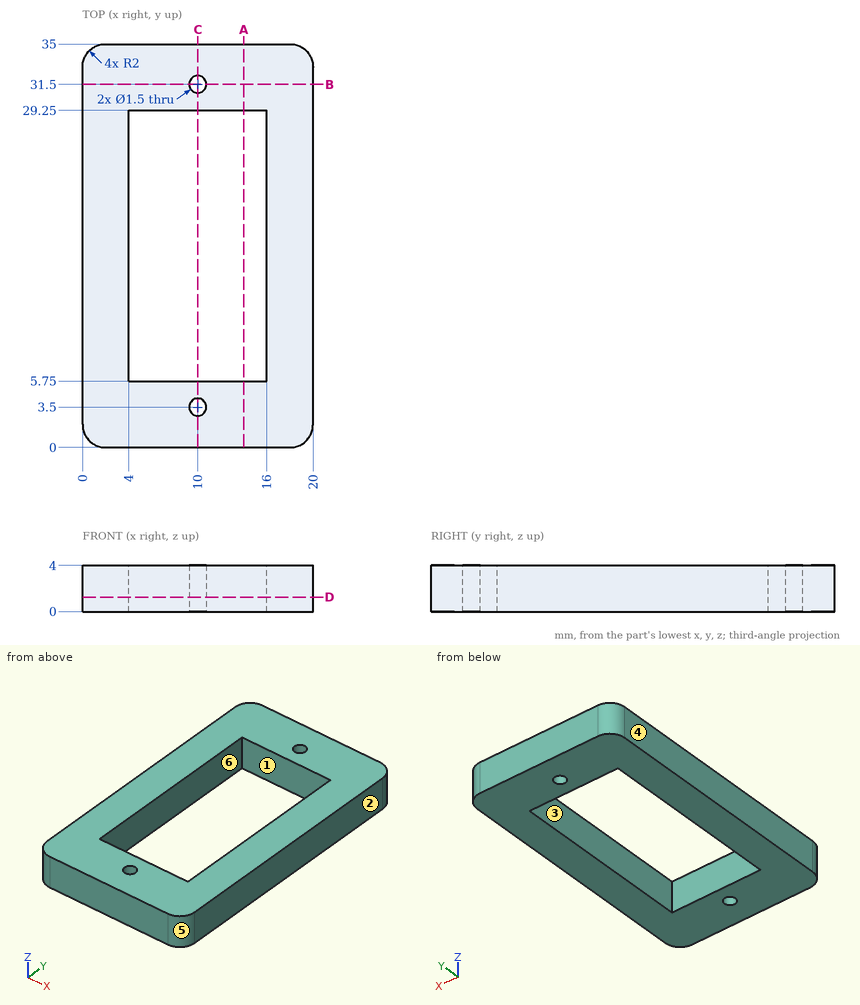
For this review, use the dimensioned drawing (mm, ordinates from the lowest corner) and the shaded views. A direction names the side the tool comes from. Round coordinates to 2 decimals unless told otherwise and drop trailing zeros. Write each loop counter-clockwise with the first axis right and the second up, starting at its lowest first coordinate (ties: lowest second). Pieces come first, ordered by that corner, then holes. Notation, with made-up numbers: (31, 62.25) -> (39, 62.25) arc R23 ccw to (39, 89.25) -> close; hole circle Ø11 at (89, 87). An arc over 180 degrees is marked (long way). Use CSV: the item, a comma, the result in double quotes.
(1) To check wall thickness, follow L1, parallel to Y at x = 10, z = 2.4; L2, parallel to Y at x = 12, z = 1.1; L3, parallel to X at y = 12, z = 2.4. State the ranges of each line that lie inside material, in increasing order. Write a range as [from, to].
Computed values:
L1,"[0, 2.75], [4.25, 5.75], [29.25, 30.75], [32.25, 35]"
L2,"[0, 5.75], [29.25, 35]"
L3,"[0, 4], [16, 20]"
(2) Consider section A-A, the plane x = 14. Give the boundary of the cut face in (y, z).
Computed values:
outline,"(0, 0) -> (5.75, 0) -> (5.75, 4) -> (0, 4) -> close; (29.25, 0) -> (35, 0) -> (35, 4) -> (29.25, 4) -> close"
(3) Clearance check with a flat-ended pin moving along its axis: P1, Ø2, axis at x = 10, y = 3.5, coming from the -Z side. State where the tip first meets the part, or that it passes through.
Computed values:
P1,"z = 0"
(4) Consider section B-B, the plane y = 31.5. Give the boundary of the cut face in (x, z).
Computed values:
outline,"(0, 0) -> (9.25, 0) -> (9.25, 4) -> (0, 4) -> close; (10.75, 0) -> (20, 0) -> (20, 4) -> (10.75, 4) -> close"
(5) For the marked faces 1 and 2, list the 3-axis set-ups (+Z, -Z, +X, -X, +Y, -Y) from which the entire face can be reached by the end or side of a thin tool; tool diameter is ignored.
Computed values:
face 1,"+Z, -Z"
face 2,"+Z, -Z, +X, +Y, -Y"
(6) Consider section D-D, the plane z = 1.25. Give the boundary of the cut face in (x, y), plus the area to 3 significant figures.
Computed values:
outline,"(0, 2) arc R2 ccw to (2, 0) -> (18, 0) arc R2 ccw to (20, 2) -> (20, 33) arc R2 ccw to (18, 35) -> (2, 35) arc R2 ccw to (0, 33) -> close; hole (4, 5.75) -> (16, 5.75) -> (16, 29.25) -> (4, 29.25) -> close; hole circle Ø1.5 at (10, 3.5); hole circle Ø1.5 at (10, 31.5)"
area,"411 mm²"
(7) Consider section C-C, the plane x = 10. Give the boundary of the cut face in (y, z).
Computed values:
outline,"(0, 0) -> (2.75, 0) -> (2.75, 4) -> (0, 4) -> close; (4.25, 0) -> (5.75, 0) -> (5.75, 4) -> (4.25, 4) -> close; (29.25, 0) -> (30.75, 0) -> (30.75, 4) -> (29.25, 4) -> close; (32.25, 0) -> (35, 0) -> (35, 4) -> (32.25, 4) -> close"
(8) Draft analysis for pull direction X (two halves, no side actions). For the marked faces 3, 4, 5 and 6, state which applies: +X half, -X half, draft (parallel to the pull), parting line (faces both ways), or undercut.
Computed values:
face 3,"undercut"
face 4,"-X half"
face 5,"+X half"
face 6,"undercut"
